from build123d import *

# Parameters (mm, degrees)
BOSS_EXTRU_1_DEPTH      = 51
ESQUISSE2_W             = 102
ESQUISSE2_H             = 122
ENL_V_MAT_EXTRU_1_DEPTH = 48
ESQUISSE4_W             = 104
ESQUISSE4_H             = 124
BOSS_EXTRU_4_DEPTH      = 1
ESQUISSE5_R             = 3
ESQUISSE5_R_2           = 1.5
BOSS_EXTRU_5_DEPTH      = 4.41
ESQUISSE7_W             = 12
ESQUISSE7_H             = 11
ENL_V_MAT_EXTRU_2_DEPTH = 3


with BuildPart() as part:
    # Esquisse1 → Boss.-Extru.1 (new body)
    with BuildSketch(Plane(origin=(0, 0, 0), x_dir=(1, 0, 0), z_dir=(0, 1, 0))):
        Polygon((0, 0), (0, 142), (3, 142), (3, 135), (108, 135), (108, 7), (3, 7), (3, 0), align=None)
    extrude(amount=BOSS_EXTRU_1_DEPTH)

    # Esquisse2 → Enlèv. mat.-Extru.1 (cut)
    with BuildSketch(Plane(origin=(0, 51, 0), x_dir=(1, 0, 0), z_dir=(0, 1, 0))):
        with Locations((54, 71)):
            Rectangle(ESQUISSE2_W, ESQUISSE2_H)
    extrude(amount=-ENL_V_MAT_EXTRU_1_DEPTH, mode=Mode.SUBTRACT)

    # Esquisse4 → Boss.-Extru.4 (add)
    with BuildSketch(Plane(origin=(0, 51, 0), x_dir=(1, 0, 0), z_dir=(0, 1, 0))):
        Polygon((1, 1), (1, 141), (2, 141), (2, 134), (107, 134), (107, 8), (2, 8), (2, 1), align=None)
        with Locations((54, 71)):
            Rectangle(ESQUISSE4_W, ESQUISSE4_H, mode=Mode.SUBTRACT)
    extrude(amount=BOSS_EXTRU_4_DEPTH)

    # Esquisse5 → Boss.-Extru.5 (add)
    # profile 1 of 8: a face of its own
    with BuildSketch(Plane(origin=(0, 3, 0), x_dir=(1, 0, 0), z_dir=(0, 1, 0))):
        with Locations(Location((74.7, 124.56, 0), (0, 0, 270))):
            Circle(ESQUISSE5_R)
        with Locations(Location((74.7, 124.56, 0), (0, 0, 270))):
            Circle(ESQUISSE5_R_2, mode=Mode.SUBTRACT)
    # profile 2 of 8: a face of its own
    with BuildSketch(Plane(origin=(0, 3, 0), x_dir=(1, 0, 0), z_dir=(0, 1, 0))):
        with Locations(Location((73.7, 74.43, 0), (0, 0, 270))):
            Circle(ESQUISSE5_R)
        with Locations(Location((73.7, 74.43, 0), (0, 0, 270))):
            Circle(ESQUISSE5_R_2, mode=Mode.SUBTRACT)
    # profile 3 of 8: a face of its own
    with BuildSketch(Plane(origin=(0, 3, 0), x_dir=(1, 0, 0), z_dir=(0, 1, 0))):
        with Locations(Location((21.9, 32.346, 0), (0, 0, 270))):
            Circle(ESQUISSE5_R)
        with Locations(Location((21.9, 32.346, 0), (0, 0, 270))):
            Circle(ESQUISSE5_R_2, mode=Mode.SUBTRACT)
    # profile 4 of 8: a face of its own
    with BuildSketch(Plane(origin=(0, 3, 0), x_dir=(1, 0, 0), z_dir=(0, 1, 0))):
        with Locations(Location((73.7, 17.456, 0), (0, 0, 270))):
            Circle(ESQUISSE5_R)
        with Locations(Location((73.7, 17.456, 0), (0, 0, 270))):
            Circle(ESQUISSE5_R_2, mode=Mode.SUBTRACT)
    # profile 5 of 8: a face of its own
    with BuildSketch(Plane(origin=(0, 3, 0), x_dir=(1, 0, 0), z_dir=(0, 1, 0))):
        with Locations(Location((21.9, 60.576, 0), (0, 0, 270))):
            Circle(ESQUISSE5_R)
        with Locations(Location((21.9, 60.576, 0), (0, 0, 270))):
            Circle(ESQUISSE5_R_2, mode=Mode.SUBTRACT)
    # profile 6 of 8: a face of its own
    with BuildSketch(Plane(origin=(0, 3, 0), x_dir=(1, 0, 0), z_dir=(0, 1, 0))):
        with Locations(Location((21.9, 119.06, 0), (0, 0, 270))):
            Circle(ESQUISSE5_R)
        with Locations(Location((21.9, 119.06, 0), (0, 0, 270))):
            Circle(ESQUISSE5_R_2, mode=Mode.SUBTRACT)
    # profile 7 of 8: a face of its own
    with BuildSketch(Plane(origin=(0, 3, 0), x_dir=(1, 0, 0), z_dir=(0, 1, 0))):
        with Locations(Location((74.7, 66.086, 0), (0, 0, 270))):
            Circle(ESQUISSE5_R)
        with Locations(Location((74.7, 66.086, 0), (0, 0, 270))):
            Circle(ESQUISSE5_R_2, mode=Mode.SUBTRACT)
    # profile 8 of 8: a face of its own
    with BuildSketch(Plane(origin=(0, 3, 0), x_dir=(1, 0, 0), z_dir=(0, 1, 0))):
        with Locations(Location((21.9, 90.83, 0), (0, 0, 270))):
            Circle(ESQUISSE5_R)
        with Locations(Location((21.9, 90.83, 0), (0, 0, 270))):
            Circle(ESQUISSE5_R_2, mode=Mode.SUBTRACT)
    extrude(amount=BOSS_EXTRU_5_DEPTH)

    # Esquisse7 → Enlèv. mat.-Extru.2 (cut)
    with BuildSketch(Plane(origin=(108, 0, 0), x_dir=(0, 0, -1), z_dir=(1, 0, 0))):
        with Locations((31.04, 15.71)):
            Rectangle(ESQUISSE7_W, ESQUISSE7_H)
        with Locations((89.53, 15.71)):
            Rectangle(ESQUISSE7_W, ESQUISSE7_H)
    extrude(amount=-ENL_V_MAT_EXTRU_2_DEPTH, mode=Mode.SUBTRACT)


solid = part.part
Geometry: final body of the model. Coordinates: model frame, mm. A direction names the side the tool comes from. Give positions to 0.01 mm unless a question says otherwise; leave off trailing zeros. Write each loop counter-clockwise with the first axis right and the second up, starting at its lowest first coordinate (ties: lowest second). Pieces come first, ordered by that corner, then holes. Notation, with made-up numbers: (20, -5) - (29, -5) arc R23 cw to (29, 29) - close; hole circle Ø8 at (15.5, 61.25). An arc over 180 degrees is marked (long way). Return JSON: item names as keys, results as strings. Group by question number.
1) Section A-A on y = 17. Return the cut outline in (x, z), plus the area to 3 significant figures.
2) Mould query, pull axis Z, two halves, no side actions, for faces 4 (the cylindrical face through (75.965, 5.174, -123.754)), 5 (the flat face through (54.2, 52, -133.5)). Classes: released by +Z, released by -Z, zero draft, split by the parting line, or undercut.
3) Set-up query: faces 1 (the flat face through (75, 3, -125)), 2 (the flat face through (107, 16, -83.53)), 3 (the flat face through (55, 0, -72)). Return all of +Z, -Z, +X, -X, +Y, -Y with unobstructed straight access to the full face (end or side cutting, diameter ignored); none if empty.
4) Section B-B on z = -54.5. Return the cut outline in (x, y), plus the area to 3 significant figures.
5) Section D-D on x = 59.5. Return the cut outline in (y, z).
6) Section C-C on y = 43.5. Return the cut outline in (x, z).
7) Line query: line 1 (X direction, y = 10.5, z = -15.5); line 2 (Z direction, x = 101, y = 7); line 3 (X direction, y = 6, z = -124). Output: solid intervals per line, ascending.
8) First-contact query: P1, Ø2, axis at x = 79.5, z = -72.5, coming from the -Y side; P2, Ø1.5, axis at x = 88.5, z = -88, coming from the +Y side; P3, Ø1.5, axis at x = 53, y = 21.5, coming from the +Z side; P4, Ø1.8, axis at x = 23.5, z = -60, coming from the +Y side. Flat tips, straight axial feed; report the tip coordinate or a pass-through.
Filled in:
{
 "1": {"outline": "(0, -142) - (3, -142) - (3, -135) - (108, -135) - (108, -95.53) - (105, -95.53) - (105, -132) - (3, -132) - (3, -10) - (105, -10) - (105, -25.04) - (108, -25.04) - (108, -7) - (3, -7) - (3, 0) - (0, 0) - close; (105, -83.53) - (108, -83.53) - (108, -37.04) - (105, -37.04) - close", "area": "1,350 mm^2"},
 "2": {"face 4": "undercut", "face 5": "zero draft"},
 "3": {"face 1": "+Y", "face 2": "+X", "face 3": "+Z, -Z, +X, -X, -Y"},
 "4": {"outline": "(0, 0) - (108, 0) - (108, 51) - (107, 51) - (107, 52) - (106, 52) - (106, 51) - (105, 51) - (105, 3) - (3, 3) - (3, 51) - (2, 51) - (2, 52) - (1, 52) - (1, 51) - (0, 51) - close", "area": "614 mm^2"},
 "5": {"outline": "(0, -135) - (51, -135) - (51, -134) - (52, -134) - (52, -133) - (51, -133) - (51, -132) - (3, -132) - (3, -10) - (51, -10) - (51, -9) - (52, -9) - (52, -8) - (51, -8) - (51, -7) - (0, -7) - close"},
 "6": {"outline": "(0, -142) - (3, -142) - (3, -135) - (108, -135) - (108, -7) - (3, -7) - (3, 0) - (0, 0) - close; hole (3, -132) - (105, -132) - (105, -10) - (3, -10) - close"},
 "7": {"line 1": "x = 0 to 3, 105 to 108", "line 2": "z = -135 to -132, -10 to -7", "line 3": "x = 0 to 3, 71.75 to 73.31, 76.09 to 77.65, 105 to 108"},
 "8": {"P1": "stops at y = 0", "P2": "stops at y = 3", "P3": "stops at z = -7", "P4": "stops at y = 7.41"}
}
